Check sheet for the modelled part. Datum: model origin and axes. Units: mm. A direction names the side the tool comes from. Give positions to 0.01 mm unless a question says otherwise; leave off trailing zeros. Order: outer loops, then holes, each group sorted by start corner. A loop starts at its lowest first (then second) coordinate and runs counter-clockwise, first axis right, second up. Notation, with made-up numbers: M 41,-35.5 L 100,-35.5 A17 ccw 100,-31.5 Z; hole C 86.5,6 d10. An arc over 180 degrees is marked long. Answer in a Markdown table with one row per item. Add a question column.
from build123d import *

# Parameters (mm, degrees)
CROQUIS1_W              = 60
CROQUIS1_H              = 40
SALIENTE_EXTRUIR1_DEPTH = 7
CROQUIS2_W              = 55
CROQUIS2_H              = 35
CORTAR_EXTRUIR1_DEPTH   = 5.5
REDONDEO1_R             = 3
CROQUIS3_R              = 1.65
CORTAR_EXTRUIR2_DEPTH   = 30.5
CROQUIS5_R              = 5
CROQUIS5_R_2            = 1.65
SALIENTE_EXTRUIR2_DEPTH = 1
CROQUIS6_R              = 3
CROQUIS6_R_2            = 1.65
SALIENTE_EXTRUIR3_DEPTH = 4.5


with BuildPart() as part:
    # Croquis1 → Saliente-Extruir1 (new body)
    with BuildSketch(Plane.XY):
        Rectangle(CROQUIS1_W, CROQUIS1_H)
    extrude(amount=SALIENTE_EXTRUIR1_DEPTH)

    # Croquis2 → Cortar-Extruir1 (cut)
    with BuildSketch(Plane.XY.offset(7)):
        Rectangle(CROQUIS2_W, CROQUIS2_H)
    extrude(amount=-CORTAR_EXTRUIR1_DEPTH, mode=Mode.SUBTRACT)

    # Redondeo1
    redondeo1_edges = [part.edges().sort_by_distance(p)[0] for p in [
        (-30, 20, 3.5),
        (30, 20, 3.5),
        (30, -20, 3.5),
        (-30, -20, 3.5),
    ]]
    fillet(redondeo1_edges, radius=REDONDEO1_R)

    # Croquis3 → Cortar-Extruir2 (cut)
    with BuildSketch(Plane(origin=(0, 0, 0), x_dir=(-1, 0, 0), z_dir=(0, 0, -1))):
        with Locations((-17.5, 10)):
            Circle(CROQUIS3_R)
        with Locations((17.5, 10)):
            Circle(CROQUIS3_R)
        with Locations((17.5, -10)):
            Circle(CROQUIS3_R)
    extrude(amount=-CORTAR_EXTRUIR2_DEPTH, mode=Mode.SUBTRACT)

    # Croquis5 → Saliente-Extruir2 (add)
    # profile 1 of 3: a face of its own
    with BuildSketch(Plane.XY.offset(1.5)):
        with Locations((-17.5, 10)):
            Circle(CROQUIS5_R)
        with Locations(Location((-17.5, 10, 0), (0, 0, 180))):
            Circle(CROQUIS5_R_2, mode=Mode.SUBTRACT)
    # profile 2 of 3: a face of its own
    with BuildSketch(Plane.XY.offset(1.5)):
        with Locations((17.5, 10)):
            Circle(CROQUIS5_R)
        with Locations(Location((17.5, 10, 0), (0, 0, 180))):
            Circle(CROQUIS5_R_2, mode=Mode.SUBTRACT)
    # profile 3 of 3: a face of its own
    with BuildSketch(Plane.XY.offset(1.5)):
        with Locations((-17.5, -10)):
            Circle(CROQUIS5_R)
        with Locations(Location((-17.5, -10, 0), (0, 0, 180))):
            Circle(CROQUIS5_R_2, mode=Mode.SUBTRACT)
    extrude(amount=SALIENTE_EXTRUIR2_DEPTH)

    # Croquis6 → Saliente-Extruir3 (add)
    # profile 1 of 3: a face of its own
    with BuildSketch(Plane.XY.offset(2.5)):
        with Locations((-17.5, 10)):
            Circle(CROQUIS6_R)
        with Locations(Location((-17.5, 10, 0), (0, 0, 180))):
            Circle(CROQUIS6_R_2, mode=Mode.SUBTRACT)
    # profile 2 of 3: a face of its own
    with BuildSketch(Plane.XY.offset(2.5)):
        with Locations((17.5, 10)):
            Circle(CROQUIS6_R)
        with Locations(Location((17.5, 10, 0), (0, 0, 180))):
            Circle(CROQUIS6_R_2, mode=Mode.SUBTRACT)
    # profile 3 of 3: a face of its own
    with BuildSketch(Plane.XY.offset(2.5)):
        with Locations((-17.5, -10)):
            Circle(CROQUIS6_R)
        with Locations(Location((-17.5, -10, 0), (0, 0, 180))):
            Circle(CROQUIS6_R_2, mode=Mode.SUBTRACT)
    extrude(amount=SALIENTE_EXTRUIR3_DEPTH)


solid = part.part
Q1. Draft check along X on faces 3 (the cylindrical face through (29.1, 19.14, 3.55)), 4 (the flat face through (0, -18, 7)), 5 (the flat face through (0, 17.5, 4)), 6 (the cylindrical face through (-29.14, -19.1, 3.55)). Enter one of: pulls with the +X half, pulls with the -X half, needs draft (parallel to the pull), parting line crosses it, or undercut.
Q2. Go/stop test with flat-tipped pins: pin 1 (10 mm diameter, centred on x = 6, y = -11, fed in from +Z); pin 2 (2 mm diameter, centred on x = -17.5, y = -10, fed in from +Z). Record where each tip stops, or that it passes through.
Q3. Cross-section at A-A (z = 5.5). Record the boundary of the cut face in (x, y), and give its area (3 significant figures).
Q4. Tool access check on faces 1 (the flat face through (0, 0, 0)), 2 (the flat face through (0, 0, 1.5)). Record the directions out of +Z, -Z, +X, -X, +Y, -Y that give a thin tool (end or side, any length) a straight path to the whole face; none if there is none.
Q5. Cross-section at B-B (x = 17.5). Record the boundary of the cut face in (y, z), and give its area (3 significant figures).
Q6. Thickness scan on probe 1 along Y at (x, z) = (-17.5, 5.25); probe 2 along Y at (x, z) = (17.5, 2.25); probe 3 along X at (y, z) = (12.5, 4.25). Record the ranges inside material, lowest first.
Q7. Cross-section at C-C (y = 10). State how many separate pieces and enclosed holes the cut face has, and give its area (3 significant figures).
Values follow:
| question | item | result |
|---|---|---|
| 1 | face 3 | pulls with the +X half |
| 1 | face 4 | needs draft |
| 1 | face 5 | undercut |
| 1 | face 6 | pulls with the -X half |
| 2 | pin 1 | z = 1.5 |
| 2 | pin 2 | through |
| 3 | outline | M -30,-17 A3 ccw -27,-20 L 27,-20 A3 ccw 30,-17 L 30,17 A3 ccw 27,20 L -27,20 A3 ccw -30,17 Z; C -17.5,-10 d6; C -17.5,10 d6; C 17.5,10 d6; hole M -27.5,-17.5 L 27.5,-17.5 L 27.5,17.5 L -27.5,17.5 Z; hole C -17.5,-10 d3.3; hole C -17.5,10 d3.3; hole C 17.5,10 d3.3 |
| 3 | area | 526 mm² |
| 4 | face 1 | -Z, +X, -X, +Y, -Y |
| 4 | face 2 | +Z |
| 5 | outline | M -20,0 L 8.35,0 L 8.35,7 L 7,7 L 7,2.5 L 5,2.5 L 5,1.5 L -17.5,1.5 L -17.5,7 L -20,7 Z; M 11.65,0 L 20,0 L 20,7 L 17.5,7 L 17.5,1.5 L 15,1.5 L 15,2.5 L 13,2.5 L 13,7 L 11.65,7 Z |
| 5 | area | 101 mm² |
| 6 | probe 1 | -20 to -17.5, -13 to -11.65, -8.35 to -7, 7 to 8.35, 11.65 to 13, 17.5 to 20 |
| 6 | probe 2 | -20 to -17.5, 5 to 8.35, 11.65 to 15, 17.5 to 20 |
| 6 | probe 3 | -30 to -27.5, -19.16 to -15.84, 15.84 to 19.16, 27.5 to 30 |
| 7 | separate pieces | 3 |
| 7 | enclosed holes | 0 |
| 7 | area | 145 mm² |
